Geometry: final body of the model. Coordinates: model frame, mm. Face numbers are marked on the shaded views. Give positions to 0.01 mm unless a question says otherwise; leave off trailing zeros. Order: outer loops, then holes, each group sorted by start corner. A loop starts at its lowest first (then second) coordinate and runs counter-clockwise, first axis right, second up. Notation, with made-up numbers: (-32.75, 28) - (12.25, 28) arc R18 ccw to (12.25, 54) - close; hole circle Ø7 at (-16, 31.25). An arc over 180 degrees is marked (long way). Write item = value, one per line. Start each with the question number.
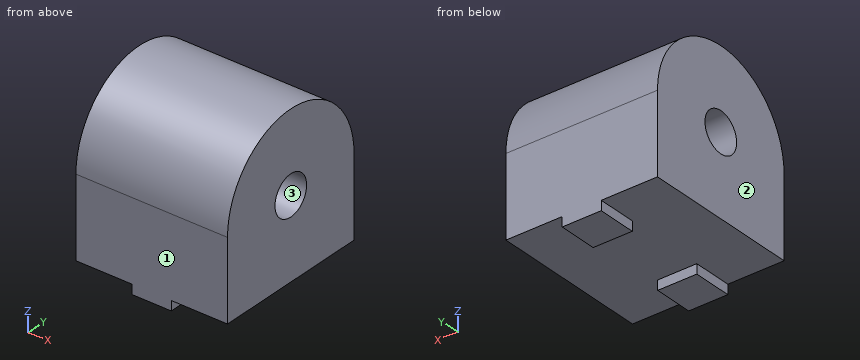
from build123d import *

# Parameters (mm, degrees)
F1_DEPTH      = 12.065
F2_W          = 6.223
F2_H          = 1.524
F3_DEPTH      = 12.7
F3_DEPTH_BACK = 12.7
F4_W          = 12.954
F4_H          = 1.524
F5_DEPTH      = 6.223


with BuildPart() as f1:
    # F0 (on Right) → F1 (new body, symmetric)
    with BuildSketch(Plane.YZ):
        with BuildLine():
            ThreePointArc((-3.175, 12.7), (0, 15.875), (3.175, 12.7))
            Line((3.175, 12.7), (12.7, 12.7))
            ThreePointArc((12.7, 12.7), (0, 25.4), (-12.7, 12.7))
            Line((-12.7, 12.7), (-3.175, 12.7))
        make_face()
        with BuildLine():
            Line((12.7, 12.7), (3.175, 12.7))
            ThreePointArc((3.175, 12.7), (0, 9.525), (-3.175, 12.7))
            Line((-3.175, 12.7), (-12.7, 12.7))
            Line((-12.7, 12.7), (-12.7, 0))
            Line((-12.7, 0), (12.7, 0))
            Line((12.7, 0), (12.7, 12.7))
        make_face()
    extrude(amount=F1_DEPTH, both=True)

    # F2 (on Front) → F3 (join, two sides)
    with BuildSketch(Plane.XZ) as f3_sk:
        with Locations((0, -0.762)):
            Rectangle(F2_W, F2_H)
    extrude(amount=F3_DEPTH)
    extrude(f3_sk.sketch, amount=-F3_DEPTH_BACK)

    # F4 (on face) → F5 (cut, through all)
    with BuildSketch(Plane(origin=(-3.1115, 0, 0), x_dir=(0, -1, 0), z_dir=(-1, 0, 0))):
        with Locations((0, -0.762)):
            Rectangle(F4_W, F4_H)
    extrude(amount=-F5_DEPTH, mode=Mode.SUBTRACT)


solid = f1.part
Q1. Contact query for flat-ended pins moving along their axis: pin 1 (7 mm diameter, centred on x = -4, y = 3, fed in from -Z); pin 2 (1.2 mm diameter, centred on y = 8, z = -1, fed in from -X); pin 3 (2 mm diameter, centred on x = 1, z = 19, fed in from +Y); pin 4 (2 mm diameter, centred on x = -4.5, y = -0.5, fed in from +Z). Output: stop coordinate, or through.
Q2. Material intervals for line 1 along Z through (x, y) = (-4, 0) (3 decimals); line 2 along Y through (x, z) = (-4, 12.7) (3 decimals); line 3 along Y through (x, z) = (-1.5, 11.5), sorted ascending. Write a range as from..to.
Q3. Section A-A, the plane x = -8.75. Return the cut outline in (y, z) (3 decimals).
Q4. Section D-D, the plane z = 18. Return the cut outline in (x, y) (3 decimals).
Q5. Section C-C, the plane y = 10.75. Return the cut outline in (x, z) (1 decimal).
Q6. Section B-B, the plane y = 0. Return the cut outline in (x, z) (3 decimals), then the cut area to 3 significant figures.
Q7. Pull-direction query (Y, two-part tool) for the marked faces 1, 2 and 3; classes: +Y half, -Y half, draft (parallel to the pull), parting line (faces both ways), or undercut.
The answers:
q1.pin_1 = 0
q1.pin_2 = -3.11
q1.pin_3 = 11.54
q1.pin_4 = 25.4
q2.line_1 = 0..9.525, 15.875..25.4
q2.line_2 = -12.7..-3.175, 3.175..12.7
q2.line_3 = -12.7..-2.94, 2.94..12.7
q3.outline = (-12.7, 0) - (12.7, 0) - (12.7, 12.7) arc R12.7 ccw to (-12.7, 12.7) - close; hole circle Ø6.35 at (0, 12.7)
q4.outline = (-12.065, -11.541) - (12.065, -11.541) - (12.065, 11.541) - (-12.065, 11.541) - close
q5.outline = (-12.1, 0) - (-3.1, 0) - (-3.1, -1.5) - (3.1, -1.5) - (3.1, 0) - (12.1, 0) - (12.1, 19.5) - (-12.1, 19.5) - close
q6.outline = (-12.065, 0) - (12.065, 0) - (12.065, 9.525) - (-12.065, 9.525) - close; (-12.065, 15.875) - (12.065, 15.875) - (12.065, 25.4) - (-12.065, 25.4) - close
q6.area = 460 mm²
q7.face_1 = -Y half
q7.face_2 = draft
q7.face_3 = undercut
